from build123d import *

# Parameters (mm, degrees)
F1_DEPTH = 35
F2_W     = 5.1841197739
F2_H     = 10
F2_R     = 1.35
F3_DEPTH = 5
F4_R     = 2.54
F5_DEPTH = 5.5
F6_DEPTH = 3.5


with BuildPart() as f1:
    # F0 (on Front) → F1 (new body)
    with BuildSketch(Plane.XZ):
        Polygon((-36.4558147092, 34.5085331884), (-36.4558147092, 19.1085331884), (-32.4558147092, 19.1085331884), (-32.4558147092, 30.5085331884), (-30.1558147092, 30.5085331884), (-30.1558147092, 12.0085331884), (-17.1558147092, 12.0085331884), (-17.1558147092, 17.0085331884), (-24.6558147092, 17.0085331884), (-24.6558147092, 34.5085331884), align=None)
    extrude(amount=F1_DEPTH)

    # F2 (on face) → F3 (join)
    with BuildSketch(Plane.XY.offset(17.0085331884)):
        with Locations((-19.7478745962, -5)):
            Rectangle(F2_W, F2_H)
        with Locations((-19.6558147092, -2.5)):
            Circle(F2_R, mode=Mode.SUBTRACT)
        with Locations((-19.7478745962, -30)):
            Rectangle(F2_W, F2_H)
        with Locations((-19.6558147092, -32.5)):
            Circle(F2_R, mode=Mode.SUBTRACT)
    extrude(amount=F3_DEPTH)

    # F4 (on face) → F5 (cut, through all)
    with BuildSketch(Plane.YZ.offset(-24.6558147092)):
        with Locations((-22.5, 24.8085331884)):
            Circle(F4_R)
        with Locations((-12.5, 24.8085331884)):
            Circle(F4_R)
    extrude(amount=-F5_DEPTH, mode=Mode.SUBTRACT)

    # F6 (cut): faces of the model
    f6_faces = [f1.faces().sort_by_distance(p)[0] for p in [
        (-19.6558147092, -32.5, 17.0085331884),
        (-19.6558147092, -2.5, 17.0085331884),
    ]]
    extrude(f6_faces, amount=-F6_DEPTH, mode=Mode.SUBTRACT)


solid = f1.part
Could you check a few things on this model? Use its own coordinates, in mm. A direction names the side the tool comes from. Round coordinates to 2 decimals unless told otherwise and drop trailing zeros. Order: outer loops, then holes, each group sorted by start corner. A loop starts at its lowest first (then second) coordinate and runs counter-clockwise, first axis right, second up. Notation, with made-up numbers: M 60.5,47 L 93.5,47 A22 ccw 93.5,69 Z; hole C 32.5,-31.75 d6. An arc over 180 degrees is marked long. One line per item, written item: value.
(1) Imagine slicing it at D-D (x = -19). Write out the boundary of the cut face in (y, z).
Ans:
outline: M -35,12.01 L 0,12.01 L 0,22.01 L -1.32,22.01 L -1.32,13.51 L -3.68,13.51 L -3.68,22.01 L -10,22.01 L -10,17.01 L -25,17.01 L -25,22.01 L -31.32,22.01 L -31.32,13.51 L -33.68,13.51 L -33.68,22.01 L -35,22.01 Z
(2) Imagine slicing it at B-B (y = -22.5). Write out the boundary of the cut face in (x, z), and give its area (3 significant figures).
Ans:
outline: M -36.46,19.11 L -32.46,19.11 L -32.46,30.51 L -30.16,30.51 L -30.16,27.35 L -24.66,27.35 L -24.66,34.51 L -36.46,34.51 Z; M -30.16,12.01 L -17.16,12.01 L -17.16,17.01 L -24.66,17.01 L -24.66,22.27 L -30.16,22.27 Z
area: 204 mm^2
(3) Which directions (+Z, -Z, +X, -X, +Y, -Y) give clear straight access to the entire face, cutting with the end or side of a thin tool? Please do faces 1 (the cylindrical face through (-27.367, -21.328, 22.555)), 2 (the flat face through (-32.456, -17, 25)), 3 (the flat face through (-20, -32, 13.509)), 4 (the flat face through (-22.34, -5, 19)), 5 (the flat face through (-34, -17, 19.109)).
Ans:
face 1: +X
face 2: -Z, +Y, -Y
face 3: +Z
face 4: +Z, +Y, -Y
face 5: -Z, -X, +Y, -Y
(4) If we mould it in two halves opening along Y, with no side actions, what happens to faces 6 (the flat face through (-24.656, -17, 26)), 7 (the flat face through (-20, -25, 19)), 8 (the flat face through (-27, -35, 23))? For each: released by +Y, released by -Y, zero draft, split by the parting line, or undercut.
Ans:
face 6: zero draft
face 7: undercut
face 8: released by -Y
(5) I need wall thicknesses on line 1 along X through (y, z) = (-33, 29.5); line 2 along Z through (x, y) = (-28.95, -22.5); line 3 along X through (y, z) = (-22.5, 23). Which ranges of each line are inside material? Lowest first, please. Write a range as from..to.
Ans:
line 1: x = -36.46..-32.46, -30.16..-24.66
line 2: z = 12.01..22.27, 27.35..34.51
line 3: x = -36.46..-32.46
(6) Imagine slicing it at A-A (z = 20.25). Write out the boundary of the cut face in (x, y).
Ans:
outline: M -36.46,-35 L -32.46,-35 L -32.46,0 L -36.46,0 Z; M -30.16,-35 L -24.66,-35 L -24.66,0 L -30.16,0 Z; M -22.34,-35 L -17.16,-35 L -17.16,-25 L -22.34,-25 Z; M -22.34,-10 L -17.16,-10 L -17.16,0 L -22.34,0 Z; hole C -19.66,-32.5 d2.7; hole C -19.66,-2.5 d2.7
(7) Imagine slicing it at C-C (z = 29.75). Write out the boundary of the cut face in (x, y), and give its area (4 significant figures).
Ans:
outline: M -36.46,-35 L -32.46,-35 L -32.46,0 L -36.46,0 Z; M -30.16,-35 L -24.66,-35 L -24.66,0 L -30.16,0 Z
area: 332.5 mm^2
(8) I'm going to push flat-ended pins straight in: P1, Ø1.6, axis at x = -19, y = -32, coming from the +Z side; P2, Ø0.8, axis at x = -20, y = -3, coming from the +Z side; P3, Ø2, axis at x = -34, y = -11.5, coming from the -Z side. Where does each tip first touch, or does it pass through?
Ans:
P1: stops at z = 22.01
P2: stops at z = 13.51
P3: stops at z = 19.11
